```python
from build123d import *

# Parameters (mm, degrees)
F0_W     = 100
F0_H     = 10
F1_DEPTH = 100
F2_DEPTH = 25
F4_DEPTH = 25
F6_DEPTH = 25


with BuildPart() as f1:
    # F0 (on Front) → F1 (new body)
    with BuildSketch(Plane.XZ):
        with Locations((25, 59.543561)):
            Rectangle(F0_W, F0_H)
    extrude(amount=F1_DEPTH)

    # F0 (on Front) → F2 (join)
    with BuildSketch(Plane.XZ):
        Polygon((-25, 54.543561), (0, 0), (50, 0), (75, 54.543561), align=None)
    extrude(amount=F2_DEPTH)

    # F3 (on face) → F4 (cut)
    with BuildSketch(Plane(origin=(0, 0, 0), x_dir=(-1, 0, 0), z_dir=(0, 1, 0))):
        with BuildLine():
            Line((-20, 17.22778), (-20, 36.596932))
            ThreePointArc((-20, 36.596932), (-25, 41.596932), (-30, 36.596932))
            Line((-30, 36.596932), (-30, 17.22778))
            ThreePointArc((-30, 17.22778), (-25, 12.22778), (-20, 17.22778))
        make_face()
    extrude(amount=-F4_DEPTH, mode=Mode.SUBTRACT)

    # F5 (on face) → F6 (cut)
    with BuildSketch(Plane.XY.offset(64.543561)):
        with BuildLine():
            Line((-5, -100), (55, -100))
            ThreePointArc((55, -100), (25, -70), (-5, -100))
        make_face()
    extrude(amount=-F6_DEPTH, mode=Mode.SUBTRACT)


solid = f1.part
```
The listing builds one solid part. Answer for the finished solid, in the listing's coordinates (mm). A direction names the side the tool comes from. Coordinates: 2 decimals unless noted, no trailing zeros. Write each loop counter-clockwise with the first axis right and the second up, starting at its lowest first coordinate (ties: lowest second). Pieces come first, ordered by that corner, then holes. Notation, with made-up numbers: (0, 75) - (6, 75) arc R14 cw to (6, 86) - close; hole circle Ø10 at (-4, 28). An arc over 180 degrees is marked (long way). Return JSON: item names as keys, results as strings. Group by question number.
Q1. The part is cut by section B-B on z = 23.5. Write down the section's boundary in (x, y).
Q2. For a pull along Z with two mould halves and no side action, classify faces 1 (the flat face through (65, -100, 60)), 2 (the cylindrical face through (25.11, -12.32, 12.23)), 3 (the flat face through (25, -12, 0)) as +Z half, -Z half, draft (parallel to the pull), parting line (faces both ways), or undercut.
Q3. Which of the six approach directions +Z, -Z, +X, -X, +Y, -Y give full straight-line access (tool end or side, diameter ignored) to faces 4 (the flat face through (62.325, -12.325, 26.89)), 5 (the flat face through (35, -25, 34)), 6 (the flat face through (20, -12, 27))?
Q4. Find the intervals of material crossed by line 1 along Z through (x, y) = (16.5, -53); line 2 along Y through (x, z) = (14, 26.5); line 3 along X through (y, z) = (-18.5, 38), in increasing order. Write a range as [from, to].
Q5. The part is cut by section D-D on y = -80. Write down the section's boundary in (x, z).
Q6. The part is cut by section A-A on y = -20.5. Write down the section's boundary in (x, z), and give its area (3 significant figures).
Q7. The part is cut by section C-C on x = 25. Write down the section's boundary in (y, z).
Q8. Flat-ended cylindrical pins translate along their axes: pin 1 Ø8 at (x, z) = (46, 24.5) entering from -Y; pin 2 Ø10 at (x, y) = (-5.5, -27) entering from -Z; pin 3 Ø21.5 at (y, z) = (-11, 26) entering from -X. Find the tip coordinate at first contact, or state that the pin passes through.
Evaluation:
{
 "1": {"outline": "(-10.77, -25) - (20, -25) - (20, 0) - (-10.77, 0) - close; (30, -25) - (60.77, -25) - (60.77, 0) - (30, 0) - close"},
 "2": {"face 1": "draft", "face 2": "undercut", "face 3": "-Z half"},
 "3": {"face 4": "-Z, +X, +Y, -Y", "face 5": "-Z, +X, -X, -Y", "face 6": "+Y, -Y"},
 "4": {"line 1": "z = [54.54, 64.54]", "line 2": "y = [-25, 0]", "line 3": "x = [-17.42, 20.2], [29.8, 67.42]"},
 "5": {"outline": "(-25, 54.54) - (2.64, 54.54) - (2.64, 64.54) - (-25, 64.54) - close; (47.36, 54.54) - (75, 54.54) - (75, 64.54) - (47.36, 64.54) - close"},
 "6": {"outline": "(-25, 54.54) - (0, 0) - (50, 0) - (75, 54.54) - (75, 64.54) - (-25, 64.54) - close; hole (20, 17.23) arc R5 ccw to (30, 17.23) - (30, 36.6) arc R5 ccw to (20, 36.6) - close", "area": "4,820 mm2"},
 "7": {"outline": "(-70, 54.54) - (-25, 54.54) - (-25, 41.6) - (0, 41.6) - (0, 64.54) - (-70, 64.54) - close; (-25, 0) - (0, 0) - (0, 12.23) - (-25, 12.23) - close"},
 "8": {"pin 1": "stops at y = -25", "pin 2": "stops at z = 2", "pin 3": "stops at x = -16.84"}
}
